Here's how the part is built. I have some questions about the finished solid (model axes, mm). A direction names the side the tool comes from. Coordinates: 2 decimals unless noted, no trailing zeros. Answer in a Markdown table with one row per item. Add a question column.
Item 1: I'm going to push flat-ended pins straight in: pin 1 (2.5 mm diameter, centred on y = 30, z = 10, fed in from +X); pin 2 (5 mm diameter, centred on y = 12, z = -14, fed in from +X); pin 3 (1.5 mm diameter, centred on y = 31, z = 6, fed in from +X); pin 4 (2.5 mm diameter, centred on y = 27, z = 11, fed in from +X). Where does each tip first touch, or does it pass through?
Item 2: Which directions (+Z, -Z, +X, -X, +Y, -Y) give clear straight access to the entire face, cutting with the end or side of a thin tool? Please do faces 1 (the face through (5.35, 26.73, -11.34)), 2 (the face through (2, 40, 0)).
Item 3: If I drill on probe 1 along Z at (x, y) = (1.2, 30); probe 2 along Y at (x, z) = (1.15, -10); probe 3 along Y at (x, z) = (13, -14), over which ranges is the centre line in solid material (lowest first)? Write a range as from..to.
Item 4: We'd pull the mould along Z, two halves only. Please class faces 3 (the face through (3, 28, -10)), 4 (the face through (0, 20, 0)), 5 (the face through (8, 11, -20)): +Z half, -Z half, draft (parallel to the pull), parting line (faces both ways), or undercut.
Item 5: Imagine slicing it at A-A (y = 30). State how many separate pieces and enclosed holes the cut face has, plus the area to 3 significant figures.
from build123d import *

# Parameters (mm, degrees)
EXTRUDE_1_DEPTH     = 20
SKETCH_2_R          = 2
CUT_EXTRUDE_2_DEPTH = 10
CUT_EXTRUDE_3_DEPTH = 20


with BuildPart() as part:
    # 草图1 → 凸台-拉伸1 (new, symmetric)
    with BuildSketch(Plane.XY):
        with BuildLine():
            Line((0, 40), (0, 0))
            Line((0, 0), (28, 0))
            Line((28, 0), (28, 4))
            add(Edge.make_bspline(
                [(28, 4), (14.27041689, 10.491058619), (2.887307451, 23.83674366), (3, 40)],
                knots=[0, 0, 0, 0, 1, 1, 1, 1], degree=3))
            Line((3, 40), (0, 40))
        make_face()
    extrude(amount=EXTRUDE_1_DEPTH, both=True)

    # 草图2 → 切除-拉伸2 (cut, symmetric)
    with BuildSketch(Plane(origin=(0, 0, 0), x_dir=(0, 0, -1), z_dir=(1, 0, 0))):
        with Locations((-10, 30)):
            Circle(SKETCH_2_R)
        with Locations((10, 30)):
            Circle(SKETCH_2_R)
    extrude(amount=CUT_EXTRUDE_2_DEPTH, both=True, mode=Mode.SUBTRACT)

    # 草图3 → 切除-拉伸3 (cut)
    with BuildSketch(Plane(origin=(5, 0, 0), x_dir=(0, 0, -1), z_dir=(1, 0, 0))):
        Polygon((-10, 34.041451884), (-13.5, 32.020725942), (-13.5, 27.979274058), (-10, 25.958548116), (-6.5, 27.979274058), (-6.5, 32.020725942), align=None)
        Polygon((10, 34.041451884), (6.5, 32.020725942), (6.5, 27.979274058), (10, 25.958548116), (13.5, 27.979274058), (13.5, 32.020725942), align=None)
    extrude(amount=CUT_EXTRUDE_3_DEPTH, mode=Mode.SUBTRACT)


solid = part.part
Here are the results:
| question | item | result |
|---|---|---|
| 1 | pin 1 | passes through |
| 1 | pin 2 | stops at x = 19.03 |
| 1 | pin 3 | stops at x = 4.36 |
| 1 | pin 4 | stops at x = 6 |
| 2 | face 1 | +X, +Y |
| 2 | face 2 | +Z, -Z, +X, -X, +Y |
| 3 | probe 1 | z = -20..-12, -8..8, 12..20 |
| 3 | probe 2 | y = 0..28, 32..40 |
| 3 | probe 3 | y = 0..15.08 |
| 4 | face 3 | undercut |
| 4 | face 4 | draft |
| 4 | face 5 | -Z half |
| 5 | separate pieces | 3 |
| 5 | enclosed holes | 0 |
| 5 | area | 142 mm2 |
